```python
from build123d import *

# Parameters (mm, degrees)
SKETCH1_R           = 6
BOSS_EXTRUDE1_DEPTH = 50
SKETCH2_R           = 17.5
BOSS_EXTRUDE2_DEPTH = 10
SKETCH3_R           = 6
BOSS_EXTRUDE3_DEPTH = 25
SKETCH4_OUTSIDE_W   = 56.672
SKETCH4_OUTSIDE_H   = 56.672
SKETCH4_OUTSIDE_W_2 = 6
SKETCH4_OUTSIDE_H_2 = 12
CUT_EXTRUDE2_DEPTH  = 8


with BuildPart() as part:
    # Sketch1 → Boss-Extrude1 (new body)
    with BuildSketch(Plane.XY):
        Circle(SKETCH1_R)
    extrude(amount=BOSS_EXTRUDE1_DEPTH)

    # Sketch2 → Boss-Extrude2 (add)
    with BuildSketch(Plane.XY.offset(50)):
        Circle(SKETCH2_R)
    extrude(amount=BOSS_EXTRUDE2_DEPTH)

    # Sketch3 → Boss-Extrude3 (add)
    with BuildSketch(Plane.XY.offset(60)):
        with Locations((0, -8)):
            Circle(SKETCH3_R)
    extrude(amount=BOSS_EXTRUDE3_DEPTH)

    # Sketch4 outside → Cut-Extrude2 (cut)
    with BuildSketch(Plane(origin=(0, 0, 0), x_dir=(-1, 0, 0), z_dir=(0, 0, -1))):
        Rectangle(SKETCH4_OUTSIDE_W, SKETCH4_OUTSIDE_H)
        Rectangle(SKETCH4_OUTSIDE_W_2, SKETCH4_OUTSIDE_H_2, mode=Mode.SUBTRACT)
    extrude(amount=-CUT_EXTRUDE2_DEPTH, mode=Mode.SUBTRACT)


solid = part.part
```
Design review of the part built by this model. Coordinates are the model's own, in mm. A direction names the side the tool comes from. Coordinates: 2 decimals unless noted, no trailing zeros. Write each loop counter-clockwise with the first axis right and the second up, starting at its lowest first coordinate (ties: lowest second). Pieces come first, ordered by that corner, then holes.
1) Machinability: for faces 1 (the cylindrical face through (-0.78, -2.05, 72.32)), 2 (the flat face through (-4, 0, 8)), 3 (the flat face through (3, 0, 4)), 4 (the flat face through (0, -8, 50)), which of the approach directions +Z, -Z, +X, -X, +Y, -Y give a long, thin tool a straight path to every point of the face, cutting with its end or side? Answer none if there is none.
2) To check wall thickness, follow L1, parallel to Z at x = 8.5, y = -2.5; L2, parallel to Z at x = 4.5, y = -1.5; L3, parallel to Y at x = 0, z = 78.5. State the ranges of each line that lie inside material, in increasing order.
3) Add section D-D (y = -8). Write out the cut boundary in (x, z).
4) Add section B-B (x = 0). Write out the cut boundary in (y, z).
5) Add section A-A (y = 0). Write out the cut boundary in (x, z).
6) Insertion check: pin 1 (6.5 mm diameter, centred on y = -2, z = 2, fed in from +X); pin 2 (9 mm diameter, centred on y = -2.5, z = 4, fed in from -X); pin 3 (3.5 mm diameter, centred on x = -4, y = 2, fed in from -Z); pin 4 (3 mm diameter, centred on y = 7, z = 20, fed in from -X). Each pin has a flat end and moves straight along its axis. Give the tip position at first contact, or say it passes through.
7) Add section C-C (z = 53.5). Write out the cut boundary in (x, y).
Check result:
1. face 1: +Z
1. face 2: -Z, -X, +Y, -Y
1. face 3: -Z, +X, +Y, -Y
1. face 4: -Z
2. L1: z = 50 to 60
2. L2: z = 8 to 60
2. L3: y = -14 to -2
3. outline: (-15.56, 50) - (15.56, 50) - (15.56, 60) - (6, 60) - (6, 85) - (-6, 85) - (-6, 60) - (-15.56, 60) - close
4. outline: (-17.5, 50) - (-6, 50) - (-6, 0) - (6, 0) - (6, 50) - (17.5, 50) - (17.5, 60) - (-2, 60) - (-2, 85) - (-14, 85) - (-14, 60) - (-17.5, 60) - close
5. outline: (-17.5, 50) - (-6, 50) - (-6, 8) - (-3, 8) - (-3, 0) - (3, 0) - (3, 8) - (6, 8) - (6, 50) - (17.5, 50) - (17.5, 60) - (-17.5, 60) - close
6. pin 1: stops at x = 3
6. pin 2: stops at x = -5.98
6. pin 3: stops at z = 0
6. pin 4: stops at x = -2.4
7. outline: circle Ø35 at (0, 0)
